Source: CAD feature listing. Evaluate the final solid. Frame: model axes, mm. Give positions to 0.01 mm unless a question says otherwise; leave off trailing zeros. Loops run counter-clockwise (first coordinate to the right, second up) from the corner with the lowest first, then second, coordinate; pieces in that order, holes last.
```python
from build123d import *

# Parameters (mm, degrees)
SKETCH_2_W          = 357
SKETCH_2_H          = 70
SKETCH_2_W_2        = 345
SKETCH_2_H_2        = 58
EXTRUDE_1_DEPTH     = 6
SKETCH_3_W          = 6
SKETCH_3_H          = 58
EXTRUDE_2_DEPTH     = 6
EXTRUDE_3_DEPTH     = 6
FILLET_1_R          = 3
SKETCH_5_W          = 6
SKETCH_5_H          = 58
EXTRUDE_4_DEPTH     = 6
EXTRUDE_5_DEPTH     = 6
FILLET_2_R          = 3
SKETCH_7_R          = 2
CUT_EXTRUDE_1_DEPTH = 6


with BuildPart() as part:
    # 草图2 → 凸台-拉伸1 (new body)
    with BuildSketch(Plane.XY):
        Rectangle(SKETCH_2_W, SKETCH_2_H)
        Rectangle(SKETCH_2_W_2, SKETCH_2_H_2, mode=Mode.SUBTRACT)
    extrude(amount=EXTRUDE_1_DEPTH)

    # 草图3 → 凸台-拉伸2 (add)
    with BuildSketch(Plane.XY):
        with Locations((-126, 0)):
            Rectangle(SKETCH_3_W, SKETCH_3_H)
        with Locations((126, 0)):
            Rectangle(SKETCH_3_W, SKETCH_3_H)
    extrude(amount=EXTRUDE_2_DEPTH)

    # 草图4 → 凸台-拉伸3 (add)
    with BuildSketch(Plane.XY):
        Polygon((-172.5, -29), (-172.5, -24), (-132.75, 29), (-129, 29), (-129, 24), (-168.75, -29), align=None)
        Polygon((129, 24), (168.75, -29), (172.5, -29), (172.5, -24), (132.75, 29), (129, 29), align=None)
    extrude(amount=EXTRUDE_3_DEPTH)

    # 圆角1
    fillet_1_edges = [part.edges().sort_by_distance(p)[0] for p in [
        (-168.75, -29, 3),
        (-129, 24, 3),
        (-132.75, 29, 3),
        (-172.5, -24, 3),
        (129, 24, 3),
        (168.75, -29, 3),
        (172.5, -24, 3),
        (132.75, 29, 3),
    ]]
    fillet(fillet_1_edges, radius=FILLET_1_R)

    # 草图5 → 凸台-拉伸4 (add)
    with BuildSketch(Plane.XY):
        with Locations((50.5, 0)):
            Rectangle(SKETCH_5_W, SKETCH_5_H)
        with Locations((-50.5, 0)):
            Rectangle(SKETCH_5_W, SKETCH_5_H)
    extrude(amount=EXTRUDE_4_DEPTH)

    # 草图6 → 凸台-拉伸5 (add)
    with BuildSketch(Plane.XY):
        Polygon((123, 29), (123, 25.092571363), (98.693529244, 4.808034617), (123, -24.317822582), (123, -29), (119.092571363, -29), (94.086919201, 0.963669401), (58.182177418, -29), (53.5, -29), (53.5, -25.092571363), (118.317822582, 29), align=None)
        Polygon((-119.092571363, -29), (-94.086919201, 0.963669401), (-58.182177418, -29), (-53.5, -29), (-53.5, -25.092571363), (-118.317822582, 29), (-123, 29), (-123, 25.092571363), (-98.693529244, 4.808034617), (-123, -24.317822582), (-123, -29), align=None)
    extrude(amount=EXTRUDE_5_DEPTH)

    # 圆角2
    fillet_2_edges = [part.edges().sort_by_distance(p)[0] for p in [
        (118.317822582, 29, 3),
        (53.5, -25.092571363, 3),
        (58.182177418, -29, 3),
        (94.086919201, 0.963669401, 3),
        (119.092571363, -29, 3),
        (123, -24.317822582, 3),
        (98.693529244, 4.808034617, 3),
        (123, 25.092571363, 3),
        (-119.092571363, -29, 3),
        (-94.086919201, 0.963669401, 3),
        (-58.182177418, -29, 3),
        (-53.5, -25.092571363, 3),
        (-118.317822582, 29, 3),
        (-123, 25.092571363, 3),
        (-98.693529244, 4.808034617, 3),
        (-123, -24.317822582, 3),
    ]]
    fillet(fillet_2_edges, radius=FILLET_2_R)

    # 草图7 → 切除-拉伸1 (cut)
    with BuildSketch(Plane(origin=(0, 0, 0), x_dir=(-1, 0, 0), z_dir=(0, 0, -1))):
        with Locations((175.5, 20)):
            Circle(SKETCH_7_R)
        with Locations((175.5, -20)):
            Circle(SKETCH_7_R)
        with Locations((50.5, 20)):
            Circle(SKETCH_7_R)
        with Locations((50.5, -20)):
            Circle(SKETCH_7_R)
        with Locations(Location((-175.5, -20, 0), (0, 0, 180))):
            Circle(SKETCH_7_R)
        with Locations(Location((-175.5, 20, 0), (0, 0, 180))):
            Circle(SKETCH_7_R)
        with Locations(Location((-50.5, -20, 0), (0, 0, 180))):
            Circle(SKETCH_7_R)
        with Locations(Location((-50.5, 20, 0), (0, 0, 180))):
            Circle(SKETCH_7_R)
        with Locations((126, 25)):
            Circle(SKETCH_7_R)
        with Locations((126, -25)):
            Circle(SKETCH_7_R)
        with Locations(Location((-126, -25, 0), (0, 0, 180))):
            Circle(SKETCH_7_R)
        with Locations(Location((-126, 25, 0), (0, 0, 180))):
            Circle(SKETCH_7_R)
    extrude(amount=-CUT_EXTRUDE_1_DEPTH, mode=Mode.SUBTRACT)


solid = part.part
```
(1) Section B-B, the plane z = 2.7. Count the separate pieces of the cut face and the enclosed holes in it, then the cut area to 3 significant figures.
A:
separate pieces: 1
enclosed holes: 23
area: 8,820 mm2
(2) Section A-A, the plane x = 75. Return the cut outline in (y, z).
A:
outline: (-35, 0) - (-29, 0) - (-29, 6) - (-35, 6) - close; (-14.96, 0) - (-7.15, 0) - (-7.15, 6) - (-14.96, 6) - close; (29, 0) - (35, 0) - (35, 6) - (29, 6) - close
(3) Ray query, line 1 along Y through (x, z) = (50.5, 1.35); line 2 along Y through (x, z) = (112, 2.35); line 3 along Y through (x, z) = (-126, 2.9). Return the intervals inside material, ascending.
A:
line 1: y = -35 to -22, -18 to 18, 22 to 35
line 2: y = -35 to -29, -20.5 to -11.14, 15.91 to 23.73, 28.27 to 35
line 3: y = -35 to -27, -23 to 23, 27 to 35
(4) Mould query, pull axis Y, two halves, no side actions, for faces 1 (the flat face through (-2, -35, 3)), 2 (the flat face through (1, -31, 6)), 3 (the flat face through (-123, 1, 3)). Classes: pulls with the +Y half, pulls with the -Y half, needs draft (parallel to the pull), parting line crosses it, or undercut.
A:
face 1: pulls with the -Y half
face 2: needs draft
face 3: undercut
